Job drawing, mm, ordinate dimensions from the low corner. One solid piece. Give positions to 0.01 mm unless a question says otherwise; leave off trailing zeros. Order: outer loops, then holes, each group sorted by start corner. A loop starts at its lowest first (then second) coordinate and runs counter-clockwise, first axis right, second up. Notation, with made-up numbers: (63, -22) - (96, -22) arc R19 ccw to (96, 5) - close; hole circle Ø2 at (-4.5, -25.75). An arc over 180 degrees is marked (long way). Use a Markdown table: item, result. Add a question column.
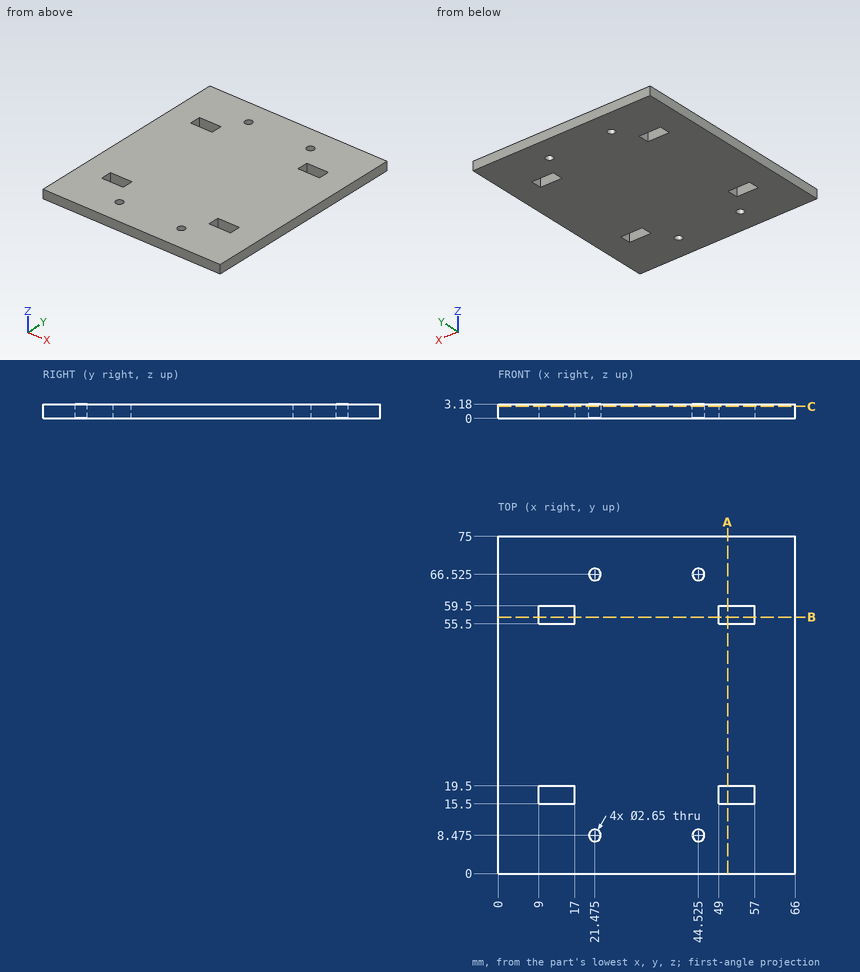
1. Pin check, flat tip, straight feed: P1, Ø2, axis at x = 21.475, y = 66.525, coming from the +Z side. Stop position of the tip, or through.
2. Cut at C-C (z = 2.65). State how many separate pieces and enclosed holes the cut face has, plus the area to 3 significant figures.
3. Cut at A-A (x = 51). Write the cut outline in (y, z), plus the area to 3 significant figures.
4. Cut at B-B (y = 57). Write the cut outline in (x, z), plus the area to 3 significant figures.
5. Drill centre line: probe 1 along X at (y, z) = (17, 2.5). Where is it in solid material? Low to high. Write a range as [from, to].
Responses:
| question | item | result |
|---|---|---|
| 1 | P1 | passes through |
| 2 | separate pieces | 1 |
| 2 | enclosed holes | 8 |
| 2 | area | 4,800 mm² |
| 3 | outline | (0, 0) - (15.5, 0) - (15.5, 3.18) - (0, 3.18) - close; (19.5, 0) - (55.5, 0) - (55.5, 3.18) - (19.5, 3.18) - close; (59.5, 0) - (75, 0) - (75, 3.18) - (59.5, 3.18) - close |
| 3 | area | 213 mm² |
| 4 | outline | (0, 0) - (9, 0) - (9, 3.18) - (0, 3.18) - close; (17, 0) - (49, 0) - (49, 3.18) - (17, 3.18) - close; (57, 0) - (66, 0) - (66, 3.18) - (57, 3.18) - close |
| 4 | area | 159 mm² |
| 5 | probe 1 | x = [0, 9], [17, 49], [57, 66] |
